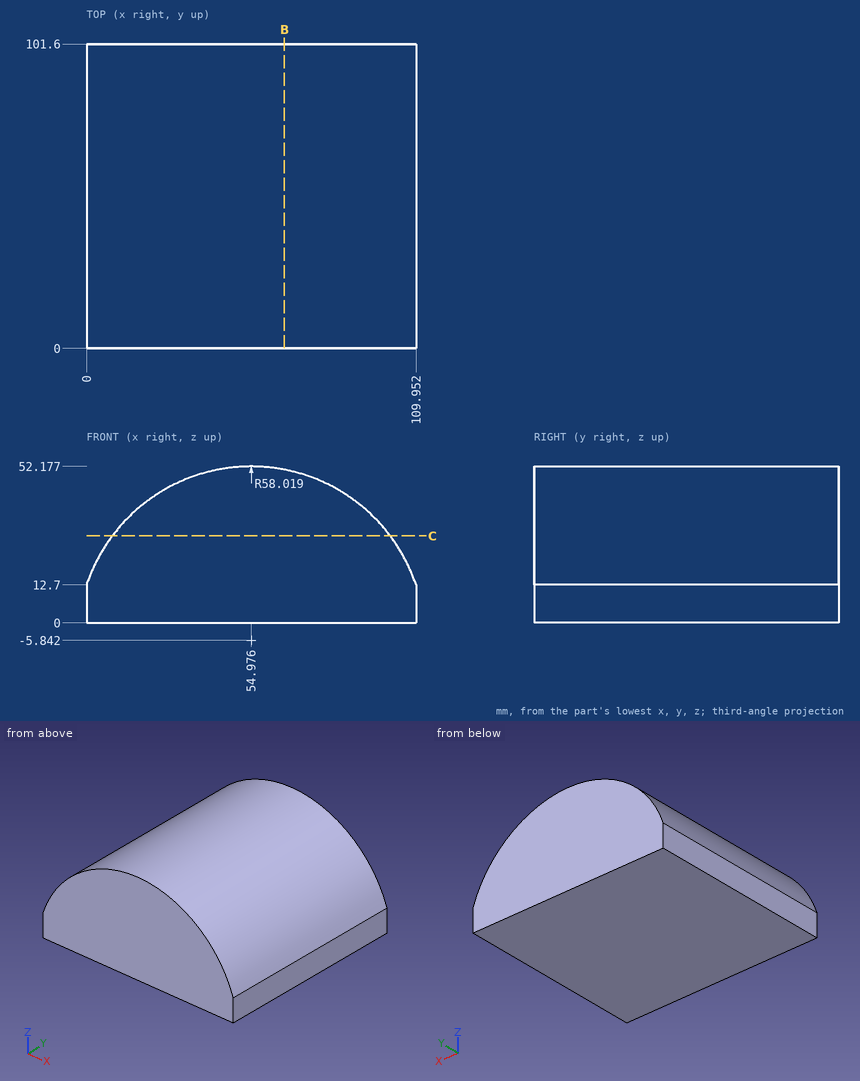
Study the drawing (mm; zero at the part's minimum x, y, z) and answer. Give positions to 0.01 mm unless a question says otherwise; leave off trailing zeros. Loops run counter-clockwise (first coordinate to the right, second up) from the corner with the lowest first, then second, coordinate; pieces in that order, holes last. Notation, with made-up numbers: (-19.5, -37.5) - (26.5, -37.5) arc R30 ccw to (26.5, -4.5) - close; hole circle Ø7 at (86, -19.5). An arc over 180 degrees is marked (long way). Answer in a Markdown table with one row per item. Add a question column.
Q1. The part is cut by section C-C (z = 29). Determine the outline of the cut face in (x, y).
Q2. Consider line 1 along X through (y, z) = (56, 14.5); line 2 along X through (y, z) = (44, 27.5) (1 decimal); line 3 along Z through (x, y) = (96, 27.5) (1 decimal). Determine where each line is inside the solid, lowest interval first.
Q3. Each of these flat-tipped pins is pushed along its axis until it touches: P1, Ø6, axis at x = 81.5, z = 35, coming from the -Y side; P2, Ø2, axis at y = 24.5, z = 27.5, coming from the +X side (1 decimal); P3, Ø8, axis at x = 60.5, y = 16.5, coming from the +Z side; P4, Ø3, axis at y = 64.5, z = 29.5, coming from the +X side. Where does it stop, or does it pass through?
Q4. The part is cut by section B-B (x = 66). Determine the outline of the cut face in (y, z).
Solution:
| question | item | result |
|---|---|---|
| 1 | outline | (8.58, 0) - (101.37, 0) - (101.37, 101.6) - (8.58, 101.6) - close |
| 2 | line 1 | x = 0.64 to 109.31 |
| 2 | line 2 | x = 7.5 to 102.5 |
| 2 | line 3 | z = 0 to 35.2 |
| 3 | P1 | stops at y = 0 |
| 3 | P2 | stops at x = 103.1 |
| 3 | P3 | stops at z = 52.16 |
| 3 | P4 | stops at x = 102.1 |
| 4 | outline | (0, 0) - (101.6, 0) - (101.6, 51.12) - (0, 51.12) - close |
